Could you check a few things on this model? Use its own coordinates, in mm. A direction names the side the tool comes from. Coordinates: 2 decimals unless noted, no trailing zeros. Order: outer loops, then holes, each group sorted by start corner. A loop starts at its lowest first (then second) coordinate and runs counter-clockwise, first axis right, second up. Notation, with made-up numbers: (-39, -25.5) -> (-32, -25.5) arc R21 ccw to (-32, -20.5) -> close; hole circle Ø11 at (66, 42.5). An arc over 180 degrees is marked (long way). Use a Markdown table: item, result. Add a question column.
1) Which directions (+Z, -Z, +X, -X, +Y, -Y) give clear straight access to the entire face, cutting with the end or side of a thin tool? Please do faces 4 (the flat face through (40, 136, -95)), 5 (the flat face through (25, 10, 0)), 6 (the flat face through (18, 91, 15)), 7 (the flat face through (25, 135, -156)), 8 (the flat face through (40, 154, -291)).
2) Thinking about a two-plate mould opening in Y: for faces 1 (the flat face through (25, 0, -20)), 2 (the cylindrical face through (45, 150, -310)), 3 (the cylindrical face through (35, -5, -17)), which applies, +Y half, -Y half, draft (parallel to the pull), parting line (faces both ways), or undercut?
3) Will these pins go through, and if not, where does the flat tip stop? pin 1 Ø5 at (x, y) = (12.5, 33.5) entering from +Z; pin 2 Ø12 at (x, y) = (33.5, 27) entering from -Z; pin 3 Ø11.5 at (x, y) = (40, -5) entering from -Z.
4) If we section it at D-D (z = -167.5): Write out the boundary of the cut face in (x, y).
5) If we section it at C-C (y = 3.5): Write out the boundary of the cut face in (x, z), plus the area to 3 significant figures.
6) If we section it at B-B (y = 150): Give the number of separate pieces and of enclosed holes in the cut face, plus the area to 3 significant figures.
7) If I drill on L1, parallel to Y at x = 42, z = -295; L2, parallel to Z at x = 21, y = -3; L3, parallel to Y at x = 17.5, z = -41.5, over which ranges is the centre line in solid material (lowest first)? Write a range as [from, to].
```python
from build123d import *

# Parameters (mm, degrees)
SKETCH1_R           = 5
BOSS_EXTRUDE1_DEPTH = 50
SKETCH2_W           = 30
SKETCH2_H           = 30
CUT_EXTRUDE1_DEPTH  = 150
SKETCH3_R           = 5
CUT_EXTRUDE2_DEPTH  = 373.323783823
FILLET1_R           = 10
FILLET2_R           = 5
FILLET3_R           = 5
SKETCH4_R           = 5
CUT_EXTRUDE3_DEPTH  = 150


with BuildPart() as part:
    # Sketch1 → Boss-Extrude1 (new body)
    with BuildSketch(Plane(origin=(0, 0, 0), x_dir=(0, 0, -1), z_dir=(1, 0, 0))):
        with BuildLine():
            Line((-15, 165), (-15, 15))
            Line((-15, 15), (-20, 15))
            Line((-20, 15), (-20, -15))
            Line((-20, -15), (-15, -15))
            Line((-15, -15), (-15, 10))
            Line((-15, 10), (15, 10))
            Line((15, 10), (15, -15))
            Line((15, -15), (20, -15))
            Line((20, -15), (20, 15))
            Line((20, 15), (15, 15))
            Line((15, 15), (15, 135))
            Line((15, 135), (295, 135))
            ThreePointArc((295, 135), (310, 150), (295, 165))
            Line((295, 165), (-15, 165))
        make_face()
        with Locations((295, 150)):
            Circle(SKETCH1_R, mode=Mode.SUBTRACT)
    extrude(amount=BOSS_EXTRUDE1_DEPTH)

    # Sketch2 → Cut-Extrude1 (cut)
    with BuildSketch(Plane(origin=(0, 165, 0), x_dir=(1, 0, 0), z_dir=(0, 1, 0))):
        with Locations((25, 295)):
            Rectangle(SKETCH2_W, SKETCH2_H)
        with BuildLine():
            Line((0, 275), (5, 275))
            ThreePointArc((5, 275), (8.535533906, 273.535533906), (10, 270))
            Line((10, 270), (10, -15))
            Line((10, -15), (0, -15))
            Line((0, -15), (0, 275))
        make_face()
        with BuildLine():
            Line((50, -15), (40, -15))
            Line((40, -15), (40, 270))
            ThreePointArc((40, 270), (41.464466094, 273.535533906), (45, 275))
            Line((45, 275), (50, 275))
            Line((50, 275), (50, -15))
        make_face()
    extrude(amount=-CUT_EXTRUDE1_DEPTH, mode=Mode.SUBTRACT)

    # Sketch3 → Cut-Extrude2 (cut, through all)
    with BuildSketch(Plane.XY.offset(20)):
        with Locations((10, -5)):
            Circle(SKETCH3_R)
        with Locations((40, -5)):
            Circle(SKETCH3_R)
    extrude(amount=-CUT_EXTRUDE2_DEPTH, mode=Mode.SUBTRACT)

    # Fillet1
    fillet1_edges = [part.edges().sort_by_distance(p)[0] for p in [
        (0, -15, -17.5),
        (50, -15, 17.5),
        (0, -15, 17.5),
        (50, -15, -17.5),
    ]]
    fillet(fillet1_edges, radius=FILLET1_R)

    # Fillet2
    fillet2_edges = [part.edges().sort_by_distance(p)[0] for p in [
        (25, 165, 15),
        (25, 135, -15),
        (25, 15, -15),
        (25, 15, 15),
        (10, 15, 0),
        (40, 15, 0),
    ]]
    fillet(fillet2_edges, radius=FILLET2_R - 0.0001)  # a hair under: the kernel refuses the full size

    # Fillet3
    fillet3_edges = [part.edges().sort_by_distance(p)[0] for p in [
        (0, 150, -275),
        (50, 150, -275),
    ]]
    fillet(fillet3_edges, radius=FILLET3_R - 0.0001)  # a hair under: the kernel refuses the full size

    # Sketch4 → Cut-Extrude3 (cut)
    with BuildSketch(Plane.XY.offset(15)):
        with Locations((25, 90)):
            Circle(SKETCH4_R)
    extrude(amount=-CUT_EXTRUDE3_DEPTH, mode=Mode.SUBTRACT)


solid = part.part
```
Answer sheet:
| question | item | result |
|---|---|---|
| 1 | face 4 | +Z, +X, +Y |
| 1 | face 5 | +X, -X, -Y |
| 1 | face 6 | +Z, +X, -X, +Y |
| 1 | face 7 | -Z, +X, -X, -Y |
| 1 | face 8 | -Z, +Y, -Y |
| 2 | face 1 | draft |
| 2 | face 2 | parting line |
| 2 | face 3 | undercut |
| 3 | pin 1 | z = 15 |
| 3 | pin 2 | z = -15 |
| 3 | pin 3 | z = -20 |
| 4 | outline | (10, 135) -> (40, 135) -> (40, 165) -> (10, 165) -> close |
| 5 | outline | (0, -20) -> (50, -20) -> (50, -15) -> (0, -15) -> close; (0, 15) -> (50, 15) -> (50, 20) -> (0, 20) -> close |
| 5 | area | 500 mm2 |
| 6 | separate pieces | 3 |
| 6 | enclosed holes | 0 |
| 6 | area | 9,350 mm2 |
| 7 | L1 | [135, 145], [155, 165] |
| 7 | L2 | [-20, -15], [15, 20] |
| 7 | L3 | [135, 165] |
